```python
from build123d import *

# Parameters (mm, degrees)
SKETCH1_W           = 11.5
SKETCH1_H           = 11.5
BOSS_EXTRUDE1_DEPTH = 195
BOSS_EXTRUDE2_START = -5.75
SKETCH2_W           = 11.5
SKETCH2_H           = 11.5
BOSS_EXTRUDE2_DEPTH = 100


with BuildPart() as part:
    # Sketch1 → Boss-Extrude1 (new body)
    with BuildSketch(Plane.XY):
        Rectangle(SKETCH1_W, SKETCH1_H)
    extrude(amount=BOSS_EXTRUDE1_DEPTH)

    # Sketch2 → Boss-Extrude2 (add)
    with BuildSketch(Plane(origin=(0, 0, 0), x_dir=(1, 0, 0), z_dir=(0, 1, 0)).offset(BOSS_EXTRUDE2_START)):
        with Locations((0, 5.75)):
            Rectangle(SKETCH2_W, SKETCH2_H)
    extrude(amount=BOSS_EXTRUDE2_DEPTH)


solid = part.part
```
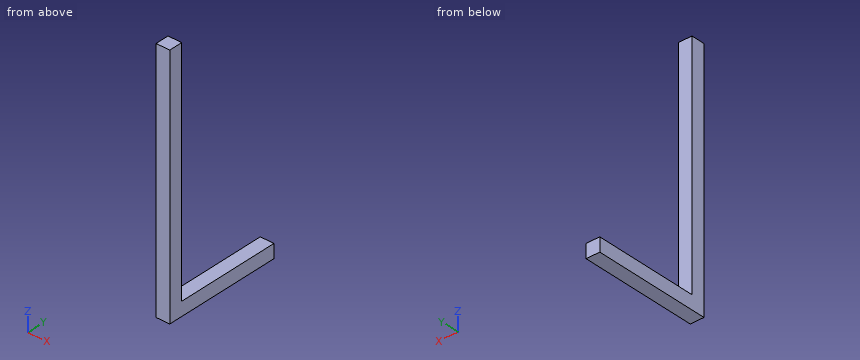
CAD build for the part. Positions are in the model's coordinates, mm. Give positions to 0.01 mm unless a question says otherwise; leave off trailing zeros. Order: outer loops, then holes, each group sorted by start corner. A loop starts at its lowest first (then second) coordinate and runs counter-clockwise, first axis right, second up.
(1) Drill centre lines: L1, parallel to Y at x = 4.5, z = 144; L2, parallel to Z at x = 3.25, y = 42.5. Where is each one in solid material? Low to high.
(2) Saw through at A-A, the plane z = 182. Give the cut face in (x, y).
(3) Saw through at C-C, the plane y = 47.5. Give the cut face in (x, z).
(4) Flat gauge pins, fed straight in: pin 1 (6 mm diameter, centred on x = -2.5, z = 86, fed in from +Y); pin 2 (2 mm diameter, centred on x = -2.5, y = 64.5, fed in from +Z). Where does each tip first touch, or does it go through?
(5) Saw through at B-B, the plane x = -2.5. Give the cut face in (y, z).
Results found:
1. L1: y = -5.75 to 5.75
1. L2: z = -11.5 to 0
2. outline: (-5.75, -5.75) - (5.75, -5.75) - (5.75, 5.75) - (-5.75, 5.75) - close
3. outline: (-5.75, -11.5) - (5.75, -11.5) - (5.75, 0) - (-5.75, 0) - close
4. pin 1: stops at y = 5.75
4. pin 2: stops at z = 0
5. outline: (-5.75, -11.5) - (94.25, -11.5) - (94.25, 0) - (5.75, 0) - (5.75, 195) - (-5.75, 195) - close
